The figure shows three views and two pictorial views of one solid part (mm, origin at its lowest corner). Answer the questions. Coordinates: 2 decimals unless noted, no trailing zeros. Order: outer loops, then holes, each group sorted by start corner. A loop starts at its lowest first (then second) coordinate and runs counter-clockwise, first axis right, second up. Notation, with made-up numbers: M 81,65 L 111,65 A8 ccw 111,69 Z; hole C -34.75,20 d5. An arc over 180 degrees is marked long. Answer in a Markdown table with one row per item. Add a question column.
Item 1: The mould has two halves that part along Z. Classify the marked faces 1 and 2: released by +Z, released by -Z, zero draft, split by the parting line, or undercut.
Item 2: The part is cut by section C-C (y = 40). Write down the section's boundary in (x, z), then the cut area to 3 significant figures.
Item 3: The part is cut by section D-D (z = 52.52). Write down the section's boundary in (x, y), then the cut area to 3 significant figures.
Item 4: The part is cut by section B-B (x = 8). Write down the section's boundary in (y, z).
Item 5: Consider line 1 (Y direction, x = 3.6, z = 88.52); line 2 (Y direction, x = 8.3, z = 88.52); line 3 (Z direction, x = 3.5, y = 27). Determine where each line is inside the solid, lowest interval first. Write a range as from..to.
Item 6: The part is cut by section A-A (z = 88.52). Write down the section's boundary in (x, y), then the cut area to 3 significant figures.
Item 7: Flat-ended cylindrical pins translate along their axes: pin 1 Ø1.5 at (x, y) = (4, 2) entering from +Z; pin 2 Ø20.5 at (y, z) = (48, 82.5) entering from +X; pin 3 Ø5 at (y, z) = (39.5, 3) entering from -X. Find the tip coordinate at first contact, or state that the pin passes through.
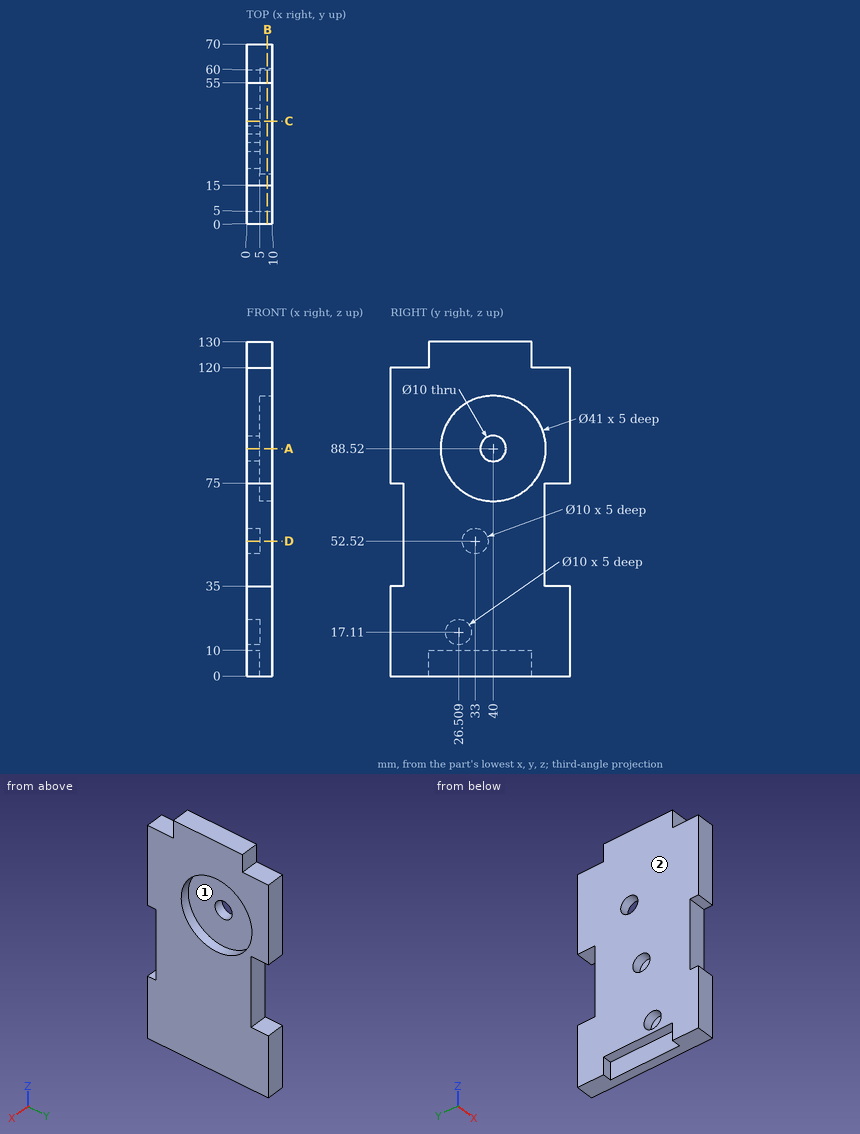
Reply:
| question | item | result |
|---|---|---|
| 1 | face 1 | undercut |
| 1 | face 2 | zero draft |
| 2 | outline | M 0,10 L 5,10 L 5,0 L 10,0 L 10,68.02 L 5,68.02 L 5,83.52 L 0,83.52 Z; M 0,93.52 L 5,93.52 L 5,109.02 L 10,109.02 L 10,130 L 0,130 Z |
| 2 | area | 995 mm2 |
| 3 | outline | M 0,5 L 10,5 L 10,60 L 0,60 L 0,38 L 5,38 L 5,28 L 0,28 Z |
| 3 | area | 500 mm2 |
| 4 | outline | M 0,0 L 70,0 L 70,35 L 60,35 L 60,75 L 70,75 L 70,120 L 55,120 L 55,130 L 15,130 L 15,120 L 0,120 L 0,75 L 5,75 L 5,35 L 0,35 Z; hole C 40,88.52 d41 |
| 5 | line 1 | y = 0..35, 45..70 |
| 5 | line 2 | y = 0..19.5, 60.5..70 |
| 5 | line 3 | z = 10..12.13, 22.09..130 |
| 6 | outline | M 0,0 L 10,0 L 10,19.5 L 5,19.5 L 5,35 L 0,35 Z; M 0,45 L 5,45 L 5,60.5 L 10,60.5 L 10,70 L 0,70 Z |
| 6 | area | 445 mm2 |
| 7 | pin 1 | stops at z = 120 |
| 7 | pin 2 | stops at x = 5 |
| 7 | pin 3 | stops at x = 5 |
